Geometry: see drawing. Coordinates: mm, zero at the bounding-box minimum. Give positions to 0.01 mm unless a question says otherwise; leave off trailing zeros. Write each loop counter-clockwise with the first axis right and the second up, starting at its lowest first coordinate (ties: lowest second). Pieces come first, ordered by that corner, then holes. Notation, with made-up numbers: (-11.75, 37) - (4.25, 37) arc R15 ccw to (4.25, 45) - close; hole circle Ø5 at (34.25, 22.25). An arc over 180 degrees is marked (long way). Use a Markdown table: item, result. Add a question column.
1. Material intervals for probe 1 along Y at (x, z) = (4, 2.6); probe 2 along X at (y, z) = (2.5, 2.6); probe 3 along X at (y, z) = (2.75, 1.15), sorted ascending.
2. Section query B-B, the plane x = 4. Return loops of the section in (y, z).
3. Mould query, pull axis Y, two halves, no side actions, for the marked faces 1, 2 and 3. Classes: released by +Y, released by -Y, zero draft, split by the parting line, or undercut.
4. Section query A-A, the plane z = 2.95. Return loops of the section in (x, y), plus the area to 3 significant figures.
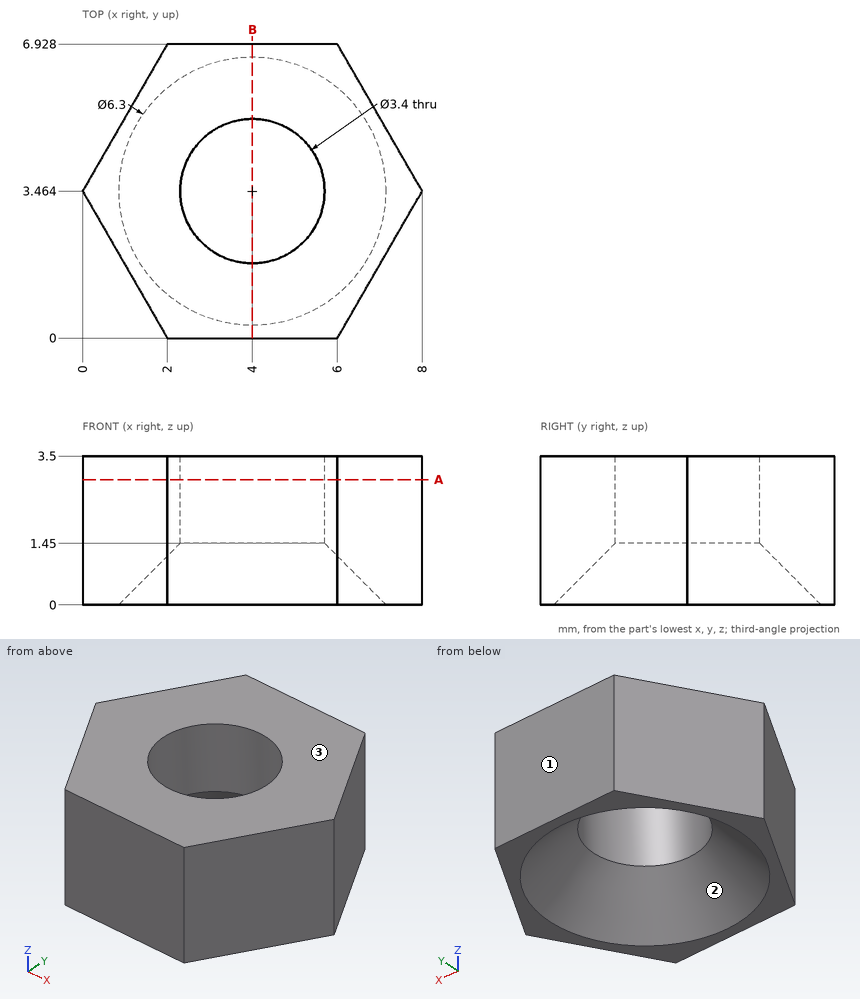
Result sheet:
| question | item | result |
|---|---|---|
| 1 | probe 1 | y = 0 to 1.76, 5.16 to 6.93 |
| 1 | probe 2 | x = 0.56 to 2.6, 5.4 to 7.44 |
| 1 | probe 3 | x = 0.41 to 2.13, 5.87 to 7.59 |
| 2 | outline | (0, 0) - (0.31, 0) - (1.76, 1.45) - (1.76, 3.5) - (0, 3.5) - close; (5.16, 1.45) - (6.61, 0) - (6.93, 0) - (6.93, 3.5) - (5.16, 3.5) - close |
| 3 | face 1 | released by +Y |
| 3 | face 2 | undercut |
| 3 | face 3 | zero draft |
| 4 | outline | (0, 3.46) - (2, 0) - (6, 0) - (8, 3.46) - (6, 6.93) - (2, 6.93) - close; hole circle Ø3.4 at (4, 3.46) |
| 4 | area | 32.5 mm² |
